from build123d import *

# Parameters (mm, degrees)
F0_W     = 177.8
F0_H     = 127
F1_DEPTH = 254
F2_R     = 25.4
F3_T     = 25.4


# Not quite as in the source:
# - a shell that OpenCascade refuses in one call is made with other operations: the cavity is built on its own and cut out


with BuildPart() as f1:
    # F0 (on Front) → F1 (new body)
    with BuildSketch(Plane.XZ):
        with Locations((118.7249161303, 53.4633891671)):
            Rectangle(F0_W, F0_H)
    extrude(amount=-F1_DEPTH)

    # F2
    f2_edges = [f1.edges().sort_by_distance(p)[0] for p in [
        (207.624916, 0, 53.463389),
        (207.624916, 254, 53.463389),
        (29.824916, 254, 53.463389),
        (29.824916, 0, 53.463389),
    ]]
    fillet(f2_edges, radius=F2_R)

    # F3: shell of thickness 25.4, made by hand


with BuildPart() as f3_core1:
    # F3_t2: copy of F1
    add(f1.part)

    # the walls: a layer under each face that stays
    f3_faces = [f3_core1.faces().sort_by_distance(p)[0] for p in [
        (207.6249161303, 127, 53.4633891671),
        (118.7249161303, 0, 53.4633891671),
        (118.7249161303, 254, 53.4633891671),
        (29.8249161303, 127, 53.4633891671),
        (118.7249161303, 127, -10.0366108329),
    ]]
    thicken(f3_faces, amount=-F3_T, mode=Mode.SUBTRACT)


with BuildPart() as f1_1:
    add(f1.part)

    # what is left inside the walls is the cavity
    f3_cavity = [f3_core1.part.solids().sort_by_distance(p)[0] for p in [
        (118.724916, 160.866667, 15.617389),
    ]]
    add(f3_cavity, mode=Mode.SUBTRACT)


solid = f1_1.part
Could you check a few things on this model? Use its own coordinates, in mm. A direction names the side the tool comes from. Give positions to 0.01 mm unless a question says otherwise; leave off trailing zeros. Order: outer loops, then holes, each group sorted by start corner. A loop starts at its lowest first (then second) coordinate and runs counter-clockwise, first axis right, second up. Notation, with made-up numbers: (2.5, -7.75) - (59.5, -7.75) arc R12 cw to (59.5, 14.25) - close; hole circle Ø9 at (79, 74). An arc over 180 degrees is marked (long way). One line per item, written item: value. Start each with the question number.
1. Imagine slicing it at C-C on z = 49.5. List the corners of the cut face in (x, y) for me.
2. For faces 1 (the face through (118, 228.6, 67)), 2 (the face through (38, 125, 116.963)), which set-ups out of +Z, -Z, +X, -X, +Y, -Y let a thin tool reach every point of the face, with its end or its side?
3. If I drill on probe 1 along Y at (x, z) = (73.5, 43.5); probe 2 along X at (y, z) = (29.5, 21); probe 3 along Y at (x, z) = (183.5, 102), over which ranges is the centre line in solid material (lowest first)?
4. For P1, Ø12, axis at x = 145.5, y = 158.5, coming from the +Z side, with a flat end and sliding along its axis, tell me the tip position at first contact or that it passes through.
5. Thinking about a two-plate mould opening in X: for faces 3 (the face through (37.068, 7.638, 54.352)), 4 (the face through (55.225, 126, 65)), 5 (the face through (200.382, 7.638, 54.352)), which applies, +X half, -X half, draft (parallel to the pull), parting line (faces both ways), or undercut?
6. Imagine slicing it at A-A on y = 88.5. List the corners of the cut face in (x, z) for me, plus the area to 3 significant figures.
7. Imagine slicing it at B-B on x = 115.5. List the corners of the cut face in (y, z) for me, plus the area to 3 significant figures.
Values:
1. outline: (29.82, 25.4) arc R25.4 ccw to (55.22, 0) - (182.22, 0) arc R25.4 ccw to (207.62, 25.4) - (207.62, 228.6) arc R25.4 ccw to (182.22, 254) - (55.22, 254) arc R25.4 ccw to (29.82, 228.6) - close; hole (55.22, 25.4) - (182.22, 25.4) - (182.22, 228.6) - (55.22, 228.6) - close
2. face 1: +Z
2. face 2: +Z, +X, -X, +Y, -Y
3. probe 1: 0 to 25.4, 228.6 to 254
3. probe 2: 29.82 to 55.22, 182.22 to 207.62
3. probe 3: 0.03 to 253.97
4. P1: z = 15.36
5. face 3: -X half
5. face 4: undercut
5. face 5: +X half
6. outline: (29.82, -10.04) - (207.62, -10.04) - (207.62, 116.96) - (182.22, 116.96) - (182.22, 15.36) - (55.22, 15.36) - (55.22, 116.96) - (29.82, 116.96) - close
6. area: 9,680 mm²
7. outline: (0, -10.04) - (254, -10.04) - (254, 116.96) - (228.6, 116.96) - (228.6, 15.36) - (25.4, 15.36) - (25.4, 116.96) - (0, 116.96) - close
7. area: 11,600 mm²
